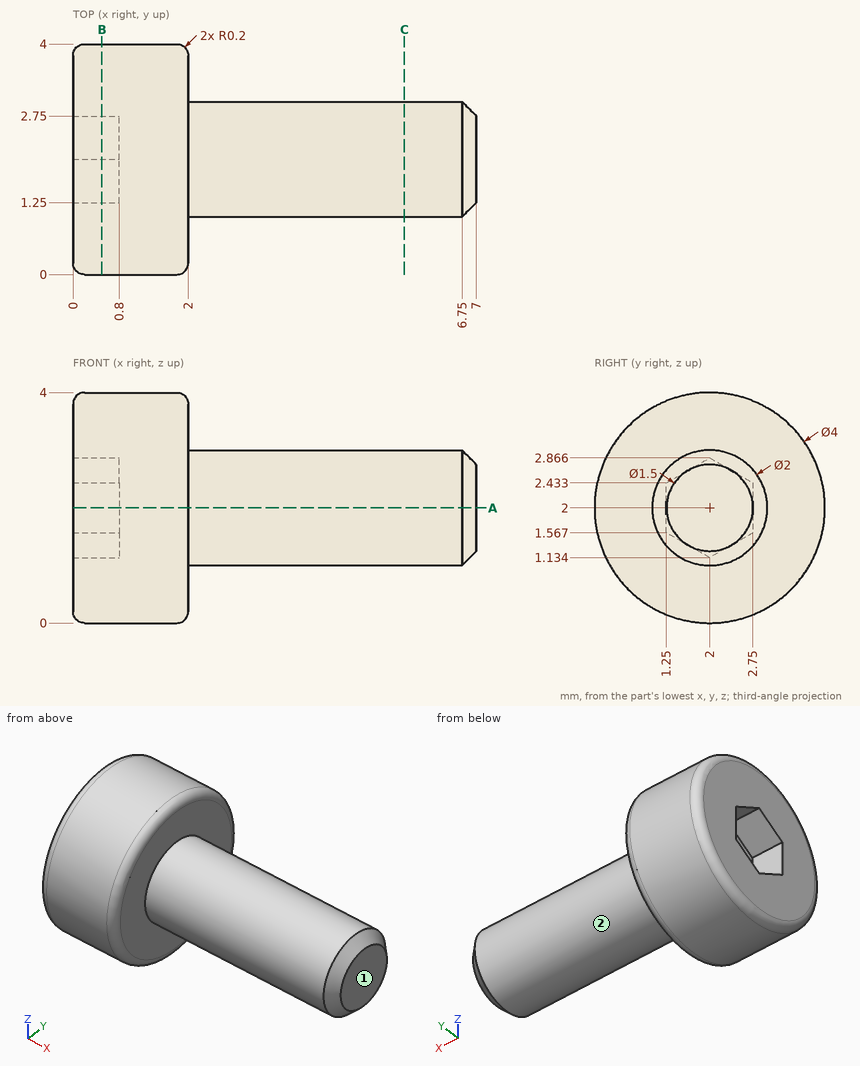
Part print with two shaded views. Sizes in mm from the minimum x, y, z corner. A direction names the side the tool comes from. Give positions to 0.01 mm unless a question says otherwise; leave off trailing zeros. Loops run counter-clockwise (first coordinate to the right, second up) from the corner with the lowest first, then second, coordinate; pieces in that order, holes last. Notation, with made-up numbers: (-35, -11.5) - (-19, -11.5) arc R19 ccw to (-19, -2.5) - close; hole circle Ø6 at (10.25, 3). An arc over 180 degrees is marked (long way). Put each result on its own line as item: value.
Q1. Slice it at C-C (x = 5.75). Give the cut face in (y, z), plus the area to 3 significant figures.
Filled in:
outline: circle Ø2 at (2, 2)
area: 3.14 mm²
Q2. Tool access for the marked faces 1 and 2: list every direction of +Z, -Z, +X, -X, +Y, -Y with a clear straight run to the whole face (end or side of a thin tool).
Filled in:
face 1: +Z, -Z, +X, +Y, -Y
face 2: +X
Q3. Flat gauge pins, fed straight in: pin 1 (1.5 mm diameter, centred on y = 3.5, z = 3.5, fed in from +X); pin 2 (1.5 mm diameter, centred on x = 3.5, z = 2, fed in from +Y). Where does each tip first touch, or does it go through?
Filled in:
pin 1: stops at x = 2
pin 2: stops at y = 3
Q4. Probe line 1 along X through (y, z) = (3.65, 2.2); line 2 along Y through (x, z) = (6.25, 2.9); line 3 along X through (y, z) = (2.25, 2.4). List the from-to ranges inside material, lowest first.
Filled in:
line 1: x = 0 to 2
line 2: y = 1.56 to 2.44
line 3: x = 0.8 to 7
Q5. Slice it at B-B (x = 0.5). Give the cut face in (y, z), plus the area to 3 significant figures.
Filled in:
outline: circle Ø4 at (2, 2); hole (1.25, 1.57) - (2, 1.13) - (2.75, 1.57) - (2.75, 2.43) - (2, 2.87) - (1.25, 2.43) - close
area: 10.6 mm²
Q6. Slice it at A-A (z = 2). Give the cut face in (x, y).
Filled in:
outline: (0, 0.2) arc R0.2 ccw to (0.2, 0) - (1.8, 0) arc R0.2 ccw to (2, 0.2) - (2, 1) - (6.75, 1) - (7, 1.25) - (7, 2.75) - (6.75, 3) - (2, 3) - (2, 3.8) arc R0.2 ccw to (1.8, 4) - (0.2, 4) arc R0.2 ccw to (0, 3.8) - (0, 2.75) - (0.8, 2.75) - (0.8, 1.25) - (0, 1.25) - close
